```python
from build123d import *

# Parameters (mm, degrees)
SKETCH1_W                = 152.4
SKETCH1_H                = 101.6
BOSS_EXTRUDE1_DEPTH      = 101.6
BOSS_EXTRUDE1_DEPTH_BACK = 5.08
SKETCH2_R                = 12.954
CUT_EXTRUDE1_DEPTH       = 101.6


with BuildPart() as part:
    # Sketch1 → Boss-Extrude1 (new body, two sides)
    with BuildSketch(Plane.XY) as boss_extrude1_sk:
        with Locations((76.2, 50.8)):
            Rectangle(SKETCH1_W, SKETCH1_H)
    extrude(amount=BOSS_EXTRUDE1_DEPTH)
    extrude(boss_extrude1_sk.sketch, amount=-BOSS_EXTRUDE1_DEPTH_BACK)

    # Sketch2 → Cut-Extrude1 (cut)
    with BuildSketch(Plane(origin=(0, 0, -5.08), x_dir=(-1, 0, 0), z_dir=(0, 0, -1))):
        with Locations((-76.2, 50.8)):
            Circle(SKETCH2_R)
    extrude(amount=-CUT_EXTRUDE1_DEPTH, mode=Mode.SUBTRACT)


solid = part.part
```
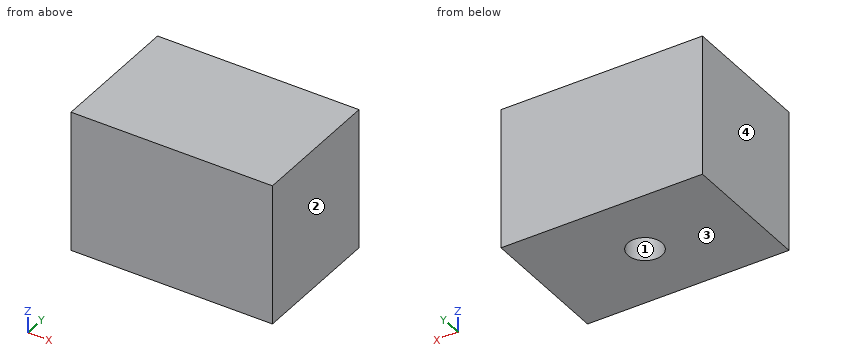
Could you check a few things on this model? Use its own coordinates, in mm. Face numbers are marked on the shaded views. Round coordinates to 2 decimals unless told otherwise and drop trailing zeros. Loops run counter-clockwise (first coordinate to the right, second up) from the corner with the lowest first, then second, coordinate; pieces in that order, holes last.
Q1. Please list where these lines run through material, in increasing order: L1, parallel to X at y = 50, z = 69; L2, parallel to Y at x = 76, z = 41; L3, parallel to Y at x = 80, z = 66.5.
Q2. Thinking about a two-plate mould opening in X: for the marked faces 1, 2, 3 and 4, which applies, pulls with the +X half, pulls with the -X half, needs draft (parallel to the pull), parting line crosses it, or undercut?
Q3. I want a section at C-C (x = 76.2). Write out the boundary of the cut face in (y, z), and give its area (3 significant figures).
Q4. I want a section at B-B (z = 89.5). Write out the boundary of the cut face in (x, y).
Q5. I want a section at A-A (y = 50.8). Write out the boundary of the cut face in (x, z), and give its area (3 significant figures).
Answer below:
1. L1: x = 0 to 63.27, 89.13 to 152.4
1. L2: y = 0 to 37.85, 63.75 to 101.6
1. L3: y = 0 to 38.42, 63.18 to 101.6
2. face 1: undercut
2. face 2: pulls with the +X half
2. face 3: needs draft
2. face 4: pulls with the -X half
3. outline: (0, -5.08) - (37.85, -5.08) - (37.85, 96.52) - (63.75, 96.52) - (63.75, -5.08) - (101.6, -5.08) - (101.6, 101.6) - (0, 101.6) - close
3. area: 8,210 mm2
4. outline: (0, 0) - (152.4, 0) - (152.4, 101.6) - (0, 101.6) - close; hole circle Ø25.91 at (76.2, 50.8)
5. outline: (0, -5.08) - (63.25, -5.08) - (63.25, 96.52) - (89.15, 96.52) - (89.15, -5.08) - (152.4, -5.08) - (152.4, 101.6) - (0, 101.6) - close
5. area: 13,600 mm2
